Geometry: see drawing. Coordinates: mm, zero at the bounding-box minimum. Coordinates: 2 decimals unless noted, no trailing zeros. Write each loop counter-clockwise with the first axis right and the second up, starting at its lowest first coordinate (ties: lowest second). Pieces come first, ordered by that corner, then holes.
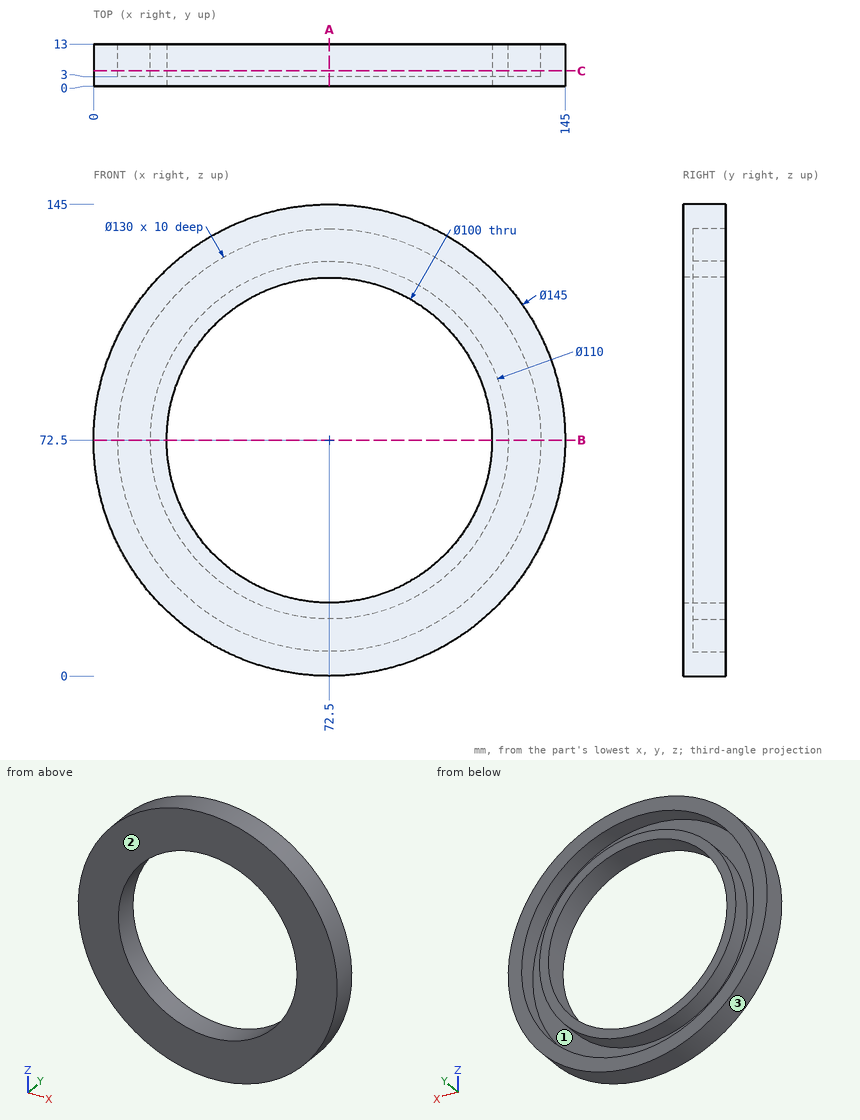
Item 1: Section C-C, the plane y = 4.75. Output: boundary loops of the cut face in (x, z), plus the area to 3 significant figures.
Derived:
outline: circle Ø145 at (72.5, 72.5); circle Ø110 at (72.5, 72.5); hole circle Ø130 at (72.5, 72.5); hole circle Ø100 at (72.5, 72.5)
area: 4,890 mm2
Item 2: Pull-direction query (X, two-part tool) for the marked faces 1, 2 and 3; classes: released by +X, released by -X, zero draft, split by the parting line, or undercut.
Derived:
face 1: undercut
face 2: zero draft
face 3: split by the parting line
Item 3: Material intervals for probe 1 along X at (y, z) = (8.75, 72.5); probe 2 along X at (y, z) = (12, 107.5); probe 3 along Z at (x, y) = (39, 6.5), sorted ascending.
Derived:
probe 1: x = 0 to 7.5, 17.5 to 22.5, 122.5 to 127.5, 137.5 to 145
probe 2: x = 9.01 to 17.73, 30.07 to 36.79, 108.21 to 114.93, 127.27 to 135.99
probe 3: z = 8.2 to 16.8, 28.88 to 35.38, 109.62 to 116.12, 128.2 to 136.8
Item 4: Section A-A, the plane x = 72.5. Output: boundary loops of the cut face in (y, z), plus the area to 3 significant figures.
Derived:
outline: (0, 0) - (13, 0) - (13, 7.5) - (3, 7.5) - (3, 17.5) - (13, 17.5) - (13, 22.5) - (0, 22.5) - close; (0, 122.5) - (13, 122.5) - (13, 127.5) - (3, 127.5) - (3, 137.5) - (13, 137.5) - (13, 145) - (0, 145) - close
area: 385 mm2
Item 5: Pin query (flat end, axial travel): pin 1 (1.5 mm diameter, centred on x = 73.5, y = 2.5, fed in from -Z); pin 2 (1.5 mm diameter, centred on x = 123.5, y = 10.5, fed in from +Z); pin 3 (6 mm diameter, centred on y = 10, z = 24.5, fed in from +X). Return the tip coordinate at first contact, or that it passes through.
Derived:
pin 1: stops at z = 0
pin 2: stops at z = 124.76
pin 3: stops at x = 129.34
Item 6: Section B-B, the plane z = 72.5. Output: boundary loops of the cut face in (x, y).
Derived:
outline: (0, 0) - (22.5, 0) - (22.5, 13) - (17.5, 13) - (17.5, 3) - (7.5, 3) - (7.5, 13) - (0, 13) - close; (122.5, 0) - (145, 0) - (145, 13) - (137.5, 13) - (137.5, 3) - (127.5, 3) - (127.5, 13) - (122.5, 13) - close
